Design review of the part built by this model. Coordinates are the model's own, in mm. A direction names the side the tool comes from. Round coordinates to 2 decimals unless told otherwise and drop trailing zeros. Loops run counter-clockwise (first coordinate to the right, second up) from the corner with the lowest first, then second, coordinate; pieces in that order, holes last. Notation, with made-up numbers: (68.25, 7) - (77.25, 7) arc R13 cw to (77.25, 32) - close; hole circle Ø1 at (62.5, -10). An arc over 180 degrees is marked (long way). One line per question, with ' | ' between items. Start each with the question number.
from build123d import *

# Parameters (mm, degrees)
PAD011_DEPTH    = 1
PAD012_DEPTH    = 17
POCKET008_DEPTH = 16
POCKET009_DEPTH = 11.6
SKETCH023_R     = 4
SKETCH023_R_2   = 1.95
SKETCH023_R_3   = 2
PAD013_DEPTH    = 5.5
SKETCH024_R     = 1.95
POCKET010_DEPTH = 8
PAD017_DEPTH    = 2.7
POCKET013_DEPTH = 17


with BuildPart() as part:
    # Sketch019 → Pad011 (new body)
    with BuildSketch(Plane.XY):
        with BuildLine():
            Line((-53.5, 45), (-53.5, -45))
            ThreePointArc((-53.5, -45), (-53.207107, -45.707107), (-52.5, -46))
            Line((-52.5, -46), (52.5, -46))
            ThreePointArc((52.5, -46), (53.207107, -45.707107), (53.5, -45))
            Line((53.5, -45), (53.5, 45))
            ThreePointArc((53.5, 45), (53.207107, 45.707107), (52.5, 46))
            Line((52.5, 46), (-52.5, 46))
            ThreePointArc((-52.5, 46), (-53.207107, 45.707107), (-53.5, 45))
        make_face()
    extrude(amount=PAD011_DEPTH)

    # Sketch020 → Pad012 (join)
    with BuildSketch(Plane.XY):
        with BuildLine():
            Line((-53.5, 45), (-53.5, -45))
            ThreePointArc((-53.5, -45), (-53.207107, -45.707107), (-52.5, -46))
            Line((-52.5, -46), (52.5, -46))
            ThreePointArc((52.5, -46), (53.207107, -45.707107), (53.5, -45))
            Line((53.5, -45), (53.5, 45))
            ThreePointArc((53.5, 45), (53.207107, 45.707107), (52.5, 46))
            Line((52.5, 46), (-52.5, 46))
            ThreePointArc((-52.5, 46), (-53.207107, 45.707107), (-53.5, 45))
        make_face()
        Polygon((-51.5, 34), (-51.5, 21.8), (-12.5, 21.8), (-12.5, -38), (51.5, -38), (51.5, 34), align=None, mode=Mode.SUBTRACT)
    extrude(amount=PAD012_DEPTH)

    # Sketch021 (on Face14 of Pad012) → Pocket008 (cut)
    with BuildSketch(Plane.XY.offset(17)):
        with BuildLine():
            Line((-52.5, 45), (-52.5, 44))
            Line((-52.5, 44), (-10, 44))
            ThreePointArc((-8.5, 42.5), (-8.93934, 43.56066), (-10, 44))
            Line((-8.5, 42.5), (-8.5, 34))
            Line((-8.5, 34), (-7, 34))
            Line((-7, 34), (-7, 42.5))
            ThreePointArc((-5.5, 44), (-6.56066, 43.56066), (-7, 42.5))
            Line((-5.5, 44), (37, 44))
            Line((37, 44), (37, 37.5))
            Line((37, 37.5), (44, 37.5))
            Line((44, 37.5), (44, 34))
            Line((45.5, 34), (44, 34))
            Line((45.5, 37.5), (45.5, 34))
            Line((45.5, 37.5), (50, 37.5))
            Line((50, 37.5), (50, 34))
            Line((50, 34), (52.5, 34))
            Line((52.5, 45), (52.5, 34))
            Line((52.5, 45), (-52.5, 45))
        make_face()
    extrude(amount=-POCKET008_DEPTH, mode=Mode.SUBTRACT)

    # Sketch022 (on Face14 of Pocket008) → Pocket009 (cut)
    with BuildSketch(Plane.XY.offset(17)):
        Polygon((-15.544, 18.358), (-51.5, 18.358), (-51.5, -38), (-15.544, -38), (-15.544, -33), (-12.5, -33), (-12.5, 13.358), (-15.544, 13.358), align=None)
    extrude(amount=-POCKET009_DEPTH, mode=Mode.SUBTRACT)

    # Sketch023 → Pad013 (join)
    with BuildSketch(Plane.XY):
        with Locations((31.5, -6)):
            Circle(SKETCH023_R)
        with Locations((31.5, -6)):
            Circle(SKETCH023_R_2, mode=Mode.SUBTRACT)
        with Locations((31.5, -28)):
            Circle(SKETCH023_R)
        with Locations((31.5, -28)):
            Circle(SKETCH023_R_2, mode=Mode.SUBTRACT)
        with Locations((0.5, -17)):
            Circle(SKETCH023_R_3)
    extrude(amount=PAD013_DEPTH)

    # Sketch024 (on Face14 of Pad013) → Pocket010 (cut)
    with BuildSketch(Plane.XY.offset(17)):
        with Locations((-49.5, -42)):
            Circle(SKETCH024_R)
        with Locations((-30, -42)):
            Circle(SKETCH024_R)
        with Locations((30, -42)):
            Circle(SKETCH024_R)
        with Locations((-49.5, 40)):
            Circle(SKETCH024_R)
        with Locations((-30, 40)):
            Circle(SKETCH024_R)
        with Locations((30, 40)):
            Circle(SKETCH024_R)
        with Locations((49.5, -42)):
            Circle(SKETCH024_R)
    extrude(amount=-POCKET010_DEPTH, mode=Mode.SUBTRACT)

    # Sketch025 (on Face4 of Pocket010) → Pad017 (join)
    with BuildSketch(Plane(origin=(0, 0, 0), x_dir=(1, 0, 0), z_dir=(0, 0, -1))):
        with BuildLine():
            Line((-50.500005, -36), (50.499995, -36))
            Line((50.499995, -36), (50.499995, 46))
            Line((52.5, 46), (50.499995, 46))
            ThreePointArc((53.5, 45), (53.207107, 45.707107), (52.5, 46))
            Line((53.5, -36), (53.5, 45))
            ThreePointArc((52.5, -37), (53.207107, -36.707107), (53.5, -36))
            Line((-52.5, -37), (52.5, -37))
            ThreePointArc((-53.5, -36), (-53.207107, -36.707107), (-52.5, -37))
            Line((-53.5, 45), (-53.5, -36))
            ThreePointArc((-52.500009, 46), (-53.20711, 45.707104), (-53.5, 45))
            Line((-52.500009, 46), (-50.500005, 46))
            Line((-50.500005, 46), (-50.500005, -36))
        make_face()
    extrude(amount=PAD017_DEPTH)

    # Sketch026 → Pocket013 (cut)
    with BuildSketch(Plane.XY):
        with BuildLine():
            ThreePointArc((-10, 0.5), (-15, -4.5), (-10, -9.5))
            Line((-10, -9.5), (10, -9.5))
            ThreePointArc((10, -9.5), (15, -4.5), (10, 0.5))
            Line((-10, 0.5), (10, 0.5))
        make_face()
    extrude(amount=POCKET013_DEPTH, mode=Mode.SUBTRACT)


solid = part.part
1. Machinability: for faces 3 (the face through (-1, 36, -1)), 4 (the face through (19, 34, 9)), 5 (the face through (-20, 21, 17)), which of the approach directions +Z, -Z, +X, -X, +Y, -Y give a long, thin tool a straight path to every point of the face, cutting with its end or side? Answer none if there is none.
2. Take a section at B-B, the plane y = -17. Give the boundary of the cut face in (x, z), then the cut area to 3 significant figures.
3. The part is to be moulded in two halves that separate along X. For faces 1 (the face through (-12.5, -26, 5)), 2 (the face through (18, 39, 17)), say which applies: pulls with the +X half, pulls with the -X half, needs draft (parallel to the pull), parting line crosses it, or undercut.
4. Take a section at A-A, the plane x = 0.5. Give the boundary of the cut face in (y, z).
5. Take a section at C-C, the plane z = 14. Count the separate pieces of the cut face and the enclosed holes in it, then the cut area to 3 significant figures.
6. Clearance check with flat-ended pins moving along their axes: P1, Ø2.5, axis at x = 30.5, y = -8, coming from the +Z side; P2, Ø5, axis at x = -3, y = 8.5, coming from the +Z side; P3, Ø6, axis at x = -30, y = -42, coming from the -Z side. State where each tip first meets the part, or that it passes through.
7. To check wall thickness, follow line 1 along Y through (x, z) = (6, 11); line 2 along Y through (x, z) = (41.5, 12.5); line 3 along Y through (x, z) = (-49.5, 12.5). State the ranges of each line that lie inside material, in increasing order.
8. Take a section at D-D, the plane x = -42. Give the boundary of the cut face in (y, z).
Answer list:
1) face 3: -Z, -Y | face 4: +Z | face 5: +Z, +X, -X, +Y, -Y
2) outline: (-53.5, -2.7) - (-50.5, -2.7) - (-50.5, 0) - (50.5, 0) - (50.5, -2.7) - (53.5, -2.7) - (53.5, 17) - (51.5, 17) - (51.5, 1) - (2.5, 1) - (2.5, 5.5) - (-1.5, 5.5) - (-1.5, 1) - (-12.5, 1) - (-12.5, 5.4) - (-51.5, 5.4) - (-51.5, 17) - (-53.5, 17) - close | area: 377 mm²
3) face 1: undercut | face 2: needs draft
4) outline: (-46, 0) - (-9.5, 0) - (-9.5, 1) - (-15, 1) - (-15, 5.5) - (-19, 5.5) - (-19, 1) - (-38, 1) - (-38, 17) - (-46, 17) - close; (0.5, 0) - (36, 0) - (36, -2.7) - (37, -2.7) - (37, 0) - (46, 0) - (46, 17) - (45, 17) - (45, 1) - (44, 1) - (44, 17) - (34, 17) - (34, 1) - (0.5, 1) - close
5) separate pieces: 3 | enclosed holes: 8 | area: 2,270 mm²
6) P1: stops at z = 5.5 | P2: stops at z = 1 | P3: stops at z = 0
7) line 1: y = -46 to -38, 34 to 44, 45 to 46 | line 2: y = -46 to -38, 34 to 37.5, 45 to 46 | line 3: y = -46 to -43.95, -40.05 to -38, 18.36 to 21.8, 34 to 38.05, 41.95 to 44, 45 to 46
8) outline: (-46, 0) - (36, 0) - (36, -2.7) - (37, -2.7) - (37, 0) - (46, 0) - (46, 17) - (45, 17) - (45, 1) - (44, 1) - (44, 17) - (34, 17) - (34, 1) - (21.8, 1) - (21.8, 17) - (18.36, 17) - (18.36, 5.4) - (-38, 5.4) - (-38, 17) - (-46, 17) - close
